Read the model definition and answer for the solid it produces. Units are mm, in the model's axes. Round coordinates to 2 decimals unless told otherwise and drop trailing zeros. Order: outer loops, then holes, each group sorted by start corner. A loop starts at its lowest first (then second) coordinate and runs counter-clockwise, first axis right, second up. Notation, with made-up numbers: (13, -15) -> (49, -15) arc R17 ccw to (49, 16) -> close; hole circle Ø5 at (35, 36.5). An arc over 180 degrees is marked (long way). One line per item, written item: value. Start each with the question number.
1. Section B-B (x = 20) is taken. Give the vertices of the cut face in (y, z).
2. The mould has two halves that part along Y. Classify faces 1 (the face through (29.4, -0.15, 3.43)), 2 (the face through (29.1, 13.14, 1.01)), 3 (the face through (17.5, 0.1, 2.3)), 4 (the face through (0, -3, 0.6)): released by +Y, released by -Y, zero draft, split by the parting line, or undercut.
3. Section D-D (x = -0.5) is taken. Give the vertices of the cut face in (y, z), then the cut area to 3 significant figures.
4. Section C-C (z = 1.35) is taken. Give the vertices of the cut face in (x, y).
5. Section A-A (y = 0) is taken. Give the vertices of the cut face in (x, z).
6. Consider line 1 (X direction, y = -2, z = 0.2); line 2 (Y direction, x = 9.5, z = 0.5); line 3 (X direction, y = 0, z = 1.35). Determine where each line is inside the solid, lowest interval first.
from build123d import *

# Parameters (mm, degrees)
F0_W     = 60
F0_H     = 28
F0_R     = 2.5
F1_DEPTH = 4
F2_W     = 54
F2_H     = 22
F3_DEPTH = 0.6
F4_R     = 3
F5_R     = 2
F6_W     = 25
F6_H     = 5
F7_DEPTH = 0.6


with BuildPart() as f1:
    # F0 (on Top) → F1 (new body)
    with BuildSketch(Plane.XY):
        Rectangle(F0_W, F0_H)
        with Locations((-20, 0)):
            Circle(F0_R, mode=Mode.SUBTRACT)
        with Locations((20, 0)):
            Circle(F0_R, mode=Mode.SUBTRACT)
    extrude(amount=F1_DEPTH)

    # F2 (on face) → F3 (cut)
    with BuildSketch(Plane(origin=(0, 0, 0), x_dir=(1, 0, 0), z_dir=(0, 0, -1))):
        Rectangle(F2_W, F2_H)
    extrude(amount=-F3_DEPTH, mode=Mode.SUBTRACT)

    # F4
    f4_edges = [f1.edges().sort_by_distance(p)[0] for p in [
        (-30, 14, 2),
        (-30, -14, 2),
        (30, -14, 2),
        (30, 14, 2),
    ]]
    fillet(f4_edges, radius=F4_R)

    # F5
    f5_edges = [f1.edges().sort_by_distance(p)[0] for p in [
        (0, 14, 4),
    ]]
    fillet(f5_edges, radius=F5_R)

    # F6 (on face) → F7 (join, through all)
    with BuildSketch(Plane(origin=(0, 0, 0.6), x_dir=(1, 0, 0), z_dir=(0, 0, -1))):
        Rectangle(F6_W, F6_H)
    extrude(amount=F7_DEPTH)


solid = f1.part
Answer:
1. outline: (-14, 0) -> (-11, 0) -> (-11, 0.6) -> (-2.5, 0.6) -> (-2.5, 4) -> (-12, 4) arc R2 ccw to (-14, 2) -> close; (2.5, 0.6) -> (11, 0.6) -> (11, 0) -> (14, 0) -> (14, 2) arc R2 ccw to (12, 4) -> (2.5, 4) -> close
2. face 1: zero draft
2. face 2: released by +Y
2. face 3: undercut
2. face 4: undercut
3. outline: (-14, 0) -> (-11, 0) -> (-11, 0.6) -> (-2.5, 0.6) -> (-2.5, 0) -> (2.5, 0) -> (2.5, 0.6) -> (11, 0.6) -> (11, 0) -> (14, 0) -> (14, 2) arc R2 ccw to (12, 4) -> (-12, 4) arc R2 ccw to (-14, 2) -> close
3. area: 100 mm^2
4. outline: (-30, -11) arc R3 ccw to (-27, -14) -> (27, -14) arc R3 ccw to (30, -11) -> (30, 11) arc R3 ccw to (27, 14) -> (-27, 14) arc R3 ccw to (-30, 11) -> close; hole circle Ø5 at (-20, 0); hole circle Ø5 at (20, 0)
5. outline: (-30, 0) -> (-27, 0) -> (-27, 0.6) -> (-22.5, 0.6) -> (-22.5, 4) -> (-28, 4) arc R2 ccw to (-30, 2) -> close; (-17.5, 0.6) -> (-12.5, 0.6) -> (-12.5, 0) -> (12.5, 0) -> (12.5, 0.6) -> (17.5, 0.6) -> (17.5, 4) -> (-17.5, 4) -> close; (22.5, 0.6) -> (27, 0.6) -> (27, 0) -> (30, 0) -> (30, 2) arc R2 ccw to (28, 4) -> (22.5, 4) -> close
6. line 1: -30 to -27, -12.5 to 12.5, 27 to 30
6. line 2: -14 to -11, -2.5 to 2.5, 11 to 14
6. line 3: -30 to -22.5, -17.5 to 17.5, 22.5 to 30
